```python
from build123d import *

# Parameters (mm, degrees)
SKETCH1_W           = 15
SKETCH1_H           = 15
BOSS_EXTRUDE1_DEPTH = 93
SKETCH2_R           = 3
BOSS_EXTRUDE2_DEPTH = 7
SKETCH3_W           = 3.2
SKETCH3_H           = 2.1
CUT_EXTRUDE1_DEPTH  = 102.396498953
FILLET1_R           = 2


with BuildPart() as part:
    # Sketch1 → Boss-Extrude1 (new body)
    with BuildSketch(Plane(origin=(0, 0, 0), x_dir=(1, 0, 0), z_dir=(0, 1, 0))):
        Rectangle(SKETCH1_W, SKETCH1_H)
    extrude(amount=BOSS_EXTRUDE1_DEPTH)

    # Sketch2 → Boss-Extrude2 (add)
    with BuildSketch(Plane(origin=(0, 93, 0), x_dir=(1, 0, 0), z_dir=(0, 1, 0))):
        with Locations(Location((1.5, 2.5, 0), (0, 0, 270))):
            Circle(SKETCH2_R)
    extrude(amount=BOSS_EXTRUDE2_DEPTH)

    # Sketch3 → Cut-Extrude1 (cut, through all)
    with BuildSketch(Plane.XY.offset(7.5)):
        with Locations((-5.9, 11.05)):
            Rectangle(SKETCH3_W, SKETCH3_H)
    extrude(amount=-CUT_EXTRUDE1_DEPTH, mode=Mode.SUBTRACT)

    # Fillet1
    fillet1_edges = [part.edges().sort_by_distance(p)[0] for p in [
        (7.5, 46.5, -7.5),
    ]]
    fillet(fillet1_edges, radius=FILLET1_R)


solid = part.part
```
Check sheet for the modelled part. Datum: model origin and axes. Units: mm. A direction names the side the tool comes from. Coordinates: 2 decimals unless noted, no trailing zeros. Loops run counter-clockwise (first coordinate to the right, second up) from the corner with the lowest first, then second, coordinate; pieces in that order, holes last.
1) Access from +Z, -Z, +X, -X, +Y, -Y to the whole of each face (thin tool, end or side, straight path). Record for faces 4 (the face through (2, 100, -3)), 5 (the face through (3.53, 96.45, -4.71)), 6 (the face through (-6, 12.1, 0)).
2) Release check for a two-part mould opening along Y. For faces 1 (the face through (6.9, 47.15, -6.93)), 2 (the face through (0, 0, 0)), 3 (the face through (-6, 10, 0)) record: released by +Y, released by -Y, zero draft, split by the parting line, or undercut.
3) Material ranges on probe 1 along Y at (x, z) = (-4.75, 6.5); probe 2 along Y at (x, z) = (-2.5, -1); probe 3 along Z at (x, y) = (6, 68.5), recorded low to high.
4) Sectioned sample at C-C (z = -2.5). Record the boundary of the cut face in (x, y).
5) Sectioned sample at A-A (z = 3.75). Record the boundary of the cut face in (x, y), and give its area (3 significant figures).
6) Sectioned sample at B-B (x = 1.5). Record the boundary of the cut face in (y, z).
7) Gauge pin test, flat end, axial feed: pin 1 (3.5 mm diameter, centred on x = -6, z = 0.5, fed in from +Y). Record the tip position at first contact, or that the pin passes through.
Check sheet entries:
1. face 4: +Z, -Z, +X, -X, +Y
1. face 5: +Y
1. face 6: +Z, -Z, -X
2. face 1: zero draft
2. face 2: released by -Y
2. face 3: undercut
3. probe 1: y = 0 to 10, 12.1 to 93
3. probe 2: y = 0 to 93
3. probe 3: z = -7.44 to 7.5
4. outline: (-7.5, 0) - (7.5, 0) - (7.5, 93) - (4.5, 93) - (4.5, 100) - (-1.5, 100) - (-1.5, 93) - (-7.5, 93) - (-7.5, 12.1) - (-4.3, 12.1) - (-4.3, 10) - (-7.5, 10) - close
5. outline: (-7.5, 0) - (7.5, 0) - (7.5, 93) - (-7.5, 93) - (-7.5, 12.1) - (-4.3, 12.1) - (-4.3, 10) - (-7.5, 10) - close
5. area: 1,390 mm2
6. outline: (0, -7.5) - (93, -7.5) - (93, -5.5) - (100, -5.5) - (100, 0.5) - (93, 0.5) - (93, 7.5) - (0, 7.5) - close
7. pin 1: stops at y = 93
